from build123d import *

# Parameters (mm, degrees)
CUT_EXTRUDE_1_DEPTH      = 3.5
CUT_EXTRUDE_1_DEPTH_BACK = 3.5
SKETCH_3_W               = 25.4
SKETCH_3_H               = 25.4


with BuildPart() as part:
    # Sketch 1 → Revolve 1 (revolve)
    with BuildSketch(Plane.XY, mode=Mode.PRIVATE) as revolve_1_sk:
        Polygon((-3.5, 0), (-3.5, 6.35), (-2.844596275, 8.796), (2.844596275, 8.796), (3.5, 6.35), (3.5, 0), align=None)
    revolve(revolve_1_sk.sketch.rotate(Axis((3.5, 0, 0), (-1, 0, 0)), 270), axis=Axis((3.5, 0, 0), (-1, 0, 0)))

    # Sketch 2 → Cut-Revolve 1 (revolve, cut)
    with BuildSketch(Plane.XY, mode=Mode.PRIVATE) as cut_revolve_1_sk:
        Polygon((-3.5, 0), (-3.5, 4), (-2.8235, 3.3235), (2.8235, 3.3235), (3.5, 4), (3.5, 0), align=None)
    revolve(cut_revolve_1_sk.sketch.rotate(Axis((3.5, 0, 0), (-1, 0, 0)), 270), axis=Axis((3.5, 0, 0), (-1, 0, 0)), mode=Mode.SUBTRACT)

    # Sketch 3 → Cut-Extrude 1 (cut, two sides: drawn at the far end of the back side and taken through both)
    with BuildSketch(Plane(origin=(0, 0, 0), x_dir=(0, 0, -1), z_dir=(1, 0, 0)).offset(-CUT_EXTRUDE_1_DEPTH_BACK)):
        Rectangle(SKETCH_3_W, SKETCH_3_H)
        Polygon((-6.35, 3.666174209), (-6.35, -3.666174209), (0, -7.332348419), (6.35, -3.666174209), (6.35, 3.666174209), (0, 7.332348419), align=None, mode=Mode.SUBTRACT)
    extrude(amount=CUT_EXTRUDE_1_DEPTH + CUT_EXTRUDE_1_DEPTH_BACK, mode=Mode.SUBTRACT)


solid = part.part
Work out the finished part from the listing and answer in its coordinate system (mm). Round coordinates to 2 decimals unless told otherwise and drop trailing zeros. Loops run counter-clockwise (first coordinate to the right, second up) from the corner with the lowest first, then second, coordinate; pieces in that order, holes last. Notation, with made-up numbers: (74, 18.5) - (88, 18.5) arc R33 ccw to (88, 55.5) - close; hole circle Ø10 at (37.25, 9.5). An arc over 180 degrees is marked (long way). One line per item, written item: value.
Q1. Straight lines are drawn through the part: probe 1 along Z at (x, y) = (-1.5, 1.75); probe 2 along Y at (x, z) = (-3, 1.75); probe 3 along Y at (x, z) = (1, 2.25). For each, find the intervals that lie inside material, in ascending order.
Check values:
probe 1: -6.35 to -2.83, 2.83 to 6.35
probe 2: -6.32 to -3.03, 3.03 to 6.32
probe 3: -6.03 to -2.45, 2.45 to 6.03
Q2. Each of these flat-tipped pins is pushed along its axis until it touches: pin 1 Ø4 at (y, z) = (3.5, -1) entering from -X; pin 2 Ø1.5 at (x, z) = (1, -4) entering from +Y; pin 3 Ø6 at (y, z) = (0, 0) entering from -X; pin 4 Ø4 at (x, z) = (0, -3.5) entering from -Y. Where does it stop, or does it pass through?
Check values:
pin 1: x = -3.5
pin 2: y = 5.46
pin 3: through
pin 4: y = -6.47
Q3. The mould has two halves that part along Y. Classify faces 1 (the flat face through (-0.049, 5.474, -3.219)), 2 (the conical face through (3.437, -3.278, -5.71)), 3 (the flat face through (-3.5, -4.1, -1.3)), 4 (the cylindrical face through (0.04, -3.244, -0.72)): +Y half, -Y half, draft (parallel to the pull), parting line (faces both ways), or undercut.
Check values:
face 1: +Y half
face 2: -Y half
face 3: draft
face 4: undercut
Q4. Find section A-A on x = -1. Give the vertices of the cut face in (y, z), and give its area (3 significant figures).
Check values:
outline: (-7.33, 0) - (-3.67, -6.35) - (3.67, -6.35) - (7.33, 0) - (3.67, 6.35) - (-3.67, 6.35) - close; hole circle Ø6.65 at (0, 0)
area: 105 mm2
